```python
from build123d import *

# Parameters (mm, degrees)
SKETCH1_W           = 25.4
SKETCH1_H           = 25.4
SKETCH1_W_2         = 22.225
SKETCH1_H_2         = 22.225
EXTRUDE_THIN1_DEPTH = 152.4
CUT_EXTRUDE1_REACH  = 27.4
SKETCH2_R           = 9.525
SKETCH2_R_2         = 1.5875
SKETCH4_R           = 3.3782
CUT_EXTRUDE2_DEPTH  = 2.5875


with BuildPart() as part:
    # Sketch1 → Extrude-Thin1 (new body)
    with BuildSketch(Plane(origin=(0, 0, 0), x_dir=(1, 0, 0), z_dir=(0, 1, 0))):
        Rectangle(SKETCH1_W, SKETCH1_H)
        Rectangle(SKETCH1_W_2, SKETCH1_H_2, mode=Mode.SUBTRACT)
    extrude(amount=EXTRUDE_THIN1_DEPTH)

    # Sketch2 → Cut-Extrude1 (cut, up to next)
    with BuildSketch(Plane.XY.offset(12.7), mode=Mode.PRIVATE) as cut_extrude1_sk1:
        with Locations((0, 114.3)):
            Circle(SKETCH2_R)
    cut_extrude1_tool1 = extrude(cut_extrude1_sk1.sketch, amount=-CUT_EXTRUDE1_REACH, mode=Mode.PRIVATE) & part.part
    add(cut_extrude1_tool1.solids().sort_by_distance((0, 114.3, 12.7))[0], mode=Mode.SUBTRACT)
    # Sketch2 → Cut-Extrude1 (cut, up to next)
    with BuildSketch(Plane.XY.offset(12.7), mode=Mode.PRIVATE) as cut_extrude1_sk2:
        with Locations((0, 38.1)):
            Circle(SKETCH2_R)
    cut_extrude1_tool2 = extrude(cut_extrude1_sk2.sketch, amount=-CUT_EXTRUDE1_REACH, mode=Mode.PRIVATE) & part.part
    add(cut_extrude1_tool2.solids().sort_by_distance((0, 38.1, 12.7))[0], mode=Mode.SUBTRACT)
    # Sketch2 → Cut-Extrude1 (cut, up to next)
    with BuildSketch(Plane.XY.offset(12.7), mode=Mode.PRIVATE) as cut_extrude1_sk3:
        with Locations((-6.35, 139.7)):
            Circle(SKETCH2_R_2)
    cut_extrude1_tool3 = extrude(cut_extrude1_sk3.sketch, amount=-CUT_EXTRUDE1_REACH, mode=Mode.PRIVATE) & part.part
    add(cut_extrude1_tool3.solids().sort_by_distance((-6.35, 139.7, 12.7))[0], mode=Mode.SUBTRACT)
    # Sketch2 → Cut-Extrude1 (cut, up to next)
    with BuildSketch(Plane.XY.offset(12.7), mode=Mode.PRIVATE) as cut_extrude1_sk4:
        with Locations((6.35, 76.2)):
            Circle(SKETCH2_R_2)
    cut_extrude1_tool4 = extrude(cut_extrude1_sk4.sketch, amount=-CUT_EXTRUDE1_REACH, mode=Mode.PRIVATE) & part.part
    add(cut_extrude1_tool4.solids().sort_by_distance((6.35, 76.2, 12.7))[0], mode=Mode.SUBTRACT)
    # Sketch2 → Cut-Extrude1 (cut, up to next)
    with BuildSketch(Plane.XY.offset(12.7), mode=Mode.PRIVATE) as cut_extrude1_sk5:
        with Locations((-6.35, 12.7)):
            Circle(SKETCH2_R_2)
    cut_extrude1_tool5 = extrude(cut_extrude1_sk5.sketch, amount=-CUT_EXTRUDE1_REACH, mode=Mode.PRIVATE) & part.part
    add(cut_extrude1_tool5.solids().sort_by_distance((-6.35, 12.7, 12.7))[0], mode=Mode.SUBTRACT)

    # Sketch4 → Cut-Extrude2 (cut, through all)
    with BuildSketch(Plane.XY.offset(-11.1125)):
        with Locations((0, 114.3)):
            Circle(SKETCH4_R)
        with Locations((0, 38.1)):
            Circle(SKETCH4_R)
    extrude(amount=-CUT_EXTRUDE2_DEPTH, mode=Mode.SUBTRACT)


solid = part.part
```
Design review of the part built by this model. Coordinates are the model's own, in mm. A direction names the side the tool comes from. Coordinates: 2 decimals unless noted, no trailing zeros. Loops run counter-clockwise (first coordinate to the right, second up) from the corner with the lowest first, then second, coordinate; pieces in that order, holes last. Notation, with made-up numbers: (28.25, -6) - (64.25, -6) arc R28 cw to (64.25, 22) - close; hole circle Ø7 at (3.25, 26). An arc over 180 degrees is marked (long way). Use CSV: the item, a comma, the result in double quotes. Start each with the question number.
1) Wall thickness on L1, parallel to Y at x = 0, z = -12.2; L2, parallel to Z at x = 2.75, y = 96; L3, parallel to X at y = 76.2, z = 11.5: over which ranges is each line inside the solid? List them lowest first. Write a range as from..to.
2) For pin 1 Ø8 at (x, y) = (0, 114.3) entering from +Z; pin 2 Ø5 at (x, z) = (8, -5) entering from -Y; pin 3 Ø4 at (x, y) = (-6.35, 12.7) entering from +Z, all flat-tipped, find the tip position at first contact; note any pin that passes through.
3) Consider section B-B on y = 114.3. Write out the cut boundary in (x, z) (1 decimal), then the cut area to 3 significant figures.
4) Consider section C-C on y = 96. Write out the cut boundary in (x, z).
5) Tool access review of faces 1 (the cylindrical face through (-0.73, 111, -11.9)), 2 (the cylindrical face through (-7.02, 120.74, 11.92)), 3 (the flat face through (0, 75, -11.112)): name each direction out of +Z, -Z, +X, -X, +Y, -Y from which nothing blocks a thin tool from reaching the whole face with its end or side.
6) The part is to be moulded in two halves that separate along Z. For faces 4 (the flat face through (-11.112, 75, 0)), 5 (the flat face through (0, 75, -12.7)), 6 (the flat face through (-11.3, 0, -0.1)), say which applies: +Z half, -Z half, draft (parallel to the pull), parting line (faces both ways), or undercut.
7) Consider section A-A on z = -1.75. Write out the cut boundary in (x, y), then the cut area to 3 significant figures.
8) Consider section D-D on x = 6.35. Write out the cut boundary in (y, z).
Geometry says:
1,L1,"0..34.72, 41.48..110.92, 117.68..152.4"
1,L2,"-12.7..-11.11, 11.11..12.7"
1,L3,"-12.7..4.76, 7.94..12.7"
2,pin 1,"z = -11.11"
2,pin 2,"through"
2,pin 3,"z = 12.7"
3,outline,"(-12.7, -12.7) - (-3.4, -12.7) - (-3.4, -11.1) - (-11.1, -11.1) - (-11.1, 11.1) - (-9.5, 11.1) - (-9.5, 12.7) - (-12.7, 12.7) - close; (3.4, -12.7) - (12.7, -12.7) - (12.7, 12.7) - (9.5, 12.7) - (9.5, 11.1) - (11.1, 11.1) - (11.1, -11.1) - (3.4, -11.1) - close"
3,area,"110 mm^2"
4,outline,"(-12.7, -12.7) - (12.7, -12.7) - (12.7, 12.7) - (-12.7, 12.7) - close; hole (-11.11, -11.11) - (11.11, -11.11) - (11.11, 11.11) - (-11.11, 11.11) - close"
5,face 1,"+Z, -Z"
5,face 2,"+Z"
5,face 3,"+Y, -Y"
6,face 4,"undercut"
6,face 5,"-Z half"
6,face 6,"draft"
7,outline,"(-12.7, 0) - (-11.11, 0) - (-11.11, 152.4) - (-12.7, 152.4) - close; (11.11, 0) - (12.7, 0) - (12.7, 152.4) - (11.11, 152.4) - close"
7,area,"484 mm^2"
8,outline,"(0, -12.7) - (152.4, -12.7) - (152.4, -11.11) - (0, -11.11) - close; (0, 11.11) - (31, 11.11) - (31, 12.7) - (0, 12.7) - close; (45.2, 11.11) - (74.61, 11.11) - (74.61, 12.7) - (45.2, 12.7) - close; (77.79, 11.11) - (107.2, 11.11) - (107.2, 12.7) - (77.79, 12.7) - close; (121.4, 11.11) - (152.4, 11.11) - (152.4, 12.7) - (121.4, 12.7) - close"
